Autodesk Inventor part; units mm, degrees
ref_plane "Work Plane1" through (5, 0, 30.15) normal (0, 0, 1) x (1, 0, 0)
ref_plane "YZ Plane" through (0, 0, 0) normal (1, 0, 0) x (0, 1, 0)
ref_plane "XZ Plane" through (0, 0, 0) normal (0, 1, 0) x (-1, 0, 0)
sketch "Sketch1" plane through (0, 0, 0) normal (0, 1, 0) x (-1, 0, 0)
  line L0 (0, 0) -> (-82, 0)
  line L1 (-82, 0) -> (-82, 60.3)
  line L2 (-82, 60.3) -> (0, 60.3)
  line L3 (0, 60.3) -> (0, 0)
  dimension "d0" = 82
  dimension "d1" = 60.3
extrude "Extrusion1" add sketch "Sketch1" along normal blind 3
sketch "Sketch3" plane through (0, 3, 0) normal (0, 1, 0) x (1, 0, 0)
  line L0 (82, -60.3) -> (82, 0)
  line L1 (82, 0) -> (0, 0)
  line L2 (21, 0) -> (61, 0)
  line L3 (61, 0) -> (61, 12)
  line L4 (61, 12) -> (21, 12)
  line L5 (21, 12) -> (21, 0)
  dimension "d22" = 82
  dimension "d23" = 12
  dimension "d24" = 21
  dimension "d25" = 40
extrude "Extrusion3" add sketch "Sketch3" against normal blind 3
sketch "Sketch4" plane through (0, 3, 0) normal (0, 1, 0) x (1, 0, 0)
  line L0 (82, 0) -> (61, 0)
  line L1 (61, 0) -> (61, 12)
  line L2 (36.5, 6.75) -> (45.5, 6.75)
  line L3 (45.5, 6.75) -> (45.5, 3.75)
  line L4 (45.5, 3.75) -> (36.5, 3.75)
  line L5 (36.5, 3.75) -> (36.5, 6.75)
  line L6 (38, 6.75) -> (43, 6.75)
  line L7 (49, 6.75) -> (51, 6.75)
  line L8 (51, 6.75) -> (51, 3.75)
  line L9 (51, 3.75) -> (49, 3.75)
  line L10 (49, 3.75) -> (49, 6.75)
  line L11 (41, 6.75) -> (41, 3.75) construction
  line L12 (33, 6.75) -> (31, 6.75)
  line L13 (31, 6.75) -> (31, 3.75)
  line L14 (31, 3.75) -> (33, 3.75)
  line L15 (33, 3.75) -> (33, 6.75)
  point P0 (21, 12)
  dimension "d28" = 9
  dimension "d29" = 3
  dimension "d30" = 3.75
  dimension "d31" = 40
  dimension "d32" = 15.5
  dimension "d42" = 2
  dimension "d43" = 3
  dimension "d44" = 3.5
extrude "Extrusion4" cut sketch "Sketch4" against normal blind 3
fillet "Fillet1" radius 5 6 edges at (0, 1.5, 60.3) (82, 1.5, 60.3) (82, 1.5, 0) (61, 1.5, -12) (21, 1.5, -12) (0, 1.5, 0)
ref_plane "Work Plane1" through (5, 0, 30.15) normal (0, 0, 1) x (1, 0, 0)
mirror "Mirror1" about plane through (5, 0, 30.15) normal (0, 0, 1) of "Extrusion3", "Extrusion4"
mirror "Mirror2" about plane through (5, 0, 30.15) normal (0, 0, 1) of "Fillet1"
equation "\"d24\" = -0.5 * d25 + 0.5 * d22"
equation "\"d32\" = -0.5 * d28 + 0.5 * d31"
properties part number "base protopress" material "Glass"
Input: part model. Units: mm. Frame: model coordinates. A direction names the side the tool comes from. Give positions to 0.01 mm unless a question says otherwise; leave off trailing zeros. Write each loop counter-clockwise with the first axis right and the second up, starting at its lowest first coordinate (ties: lowest second). Pieces come first, ordered by that corner, then holes. Notation, with made-up numbers: (47.5, -8.75) - (101.5, -8.75) arc R20 cw to (101.5, 6.25) - close; hole circle Ø10 at (70.25, 34.25). An arc over 180 degrees is marked (long way). Write item = value, one per line. Start each with the question number.
1. Ray query, L1, parallel to X at y = 0.25, z = 64.5; L2, parallel to Z at x = 5.5, y = 2.5; L3, parallel to X at y = 1.8, z = -8.5. Return the intervals inside material, ascending.
2. First-contact query: pin 1 Ø0.9 at (x, y) = (16, 1) entering from +Z; pin 2 Ø1.5 at (y, z) = (1.5, 66) entering from -X; pin 3 Ø1.5 at (y, z) = (1, -5) entering from +X; pin 4 Ø2 at (x, z) = (21, 55.5) entering from -Y. Flat tips, straight axial feed; report the tip coordinate or a pass-through.
3. Section query B-B, the plane x = 38.5. Output: boundary loops of the cut face in (y, z).
4. Section query D-D, the plane x = 63. Output: boundary loops of the cut face in (y, z).
5. Mould query, pull axis Z, two halves, no side actions, for faces 4 (the flat face through (61, 2, 64)), 5 (the flat face through (13, 1, 0)), 6 (the flat face through (49, 2, -5)). Classes: released by +Z, released by -Z, zero draft, split by the parting line, or undercut.
6. Section query A-A, the plane z = 65. Output: boundary loops of the cut face in (x, y).
7. Section query C-C, the plane y = 2.5. Count the separate pieces of the cut face and the enclosed holes in it, then the cut area to 3 significant figures.
8. Access query for faces 1 (the flat face through (13, 1, 60.3)), 2 (the flat face through (33, 2, -5)), 3 (the flat face through (82, 1, 30)). Directions: +Z, -Z, +X, -X, +Y, -Y. A direction counts if a zero-diameter tool reaches every point of the face in a straight line with its end or side. Return the directions, or none.
Check sheet entries:
q1.L1 = 21 to 31, 33 to 36.5, 45.5 to 49, 51 to 61
q1.L2 = 0 to 60.3
q1.L3 = 21.23 to 60.77
q2.pin_1 = 60.3
q2.pin_2 = 21
q2.pin_3 = 61
q2.pin_4 = 0
q3.outline = (0, -12) - (3, -12) - (3, -6.75) - (0, -6.75) - close; (0, -3.75) - (3, -3.75) - (3, 64.05) - (0, 64.05) - close; (0, 67.05) - (3, 67.05) - (3, 72.3) - (0, 72.3) - close
q4.outline = (0, 0) - (3, 0) - (3, 60.3) - (0, 60.3) - close
q5.face_4 = zero draft
q5.face_5 = released by -Z
q5.face_6 = undercut
q6.outline = (21, 0) - (31, 0) - (31, 3) - (21, 3) - close; (33, 0) - (36.5, 0) - (36.5, 3) - (33, 3) - close; (45.5, 0) - (49, 0) - (49, 3) - (45.5, 3) - close; (51, 0) - (61, 0) - (61, 3) - (51, 3) - close
q7.separate_pieces = 1
q7.enclosed_holes = 6
q7.area = 5,780 mm2
q8.face_1 = +Z, -X, +Y, -Y
q8.face_2 = +Y, -Y
q8.face_3 = +Z, -Z, +X, +Y, -Y
